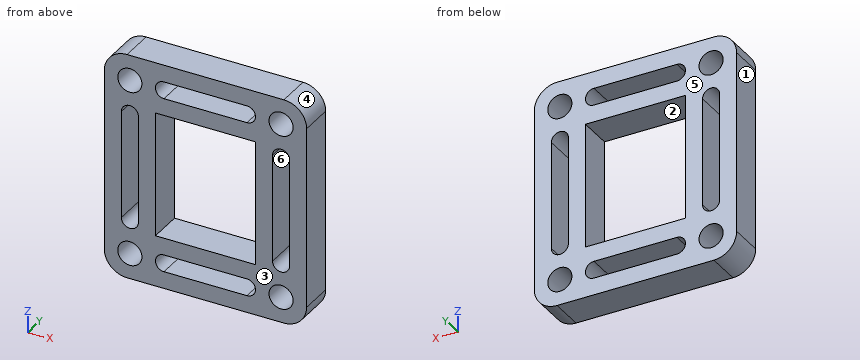
```python
from build123d import *

# Parameters (mm, degrees)
SKETCH1_R           = 2.694076836
SKETCH1_W           = 22.352
SKETCH1_H           = 27.94
BOSS_EXTRUDE1_DEPTH = 7.62


with BuildPart() as part:
    # Sketch1 → Boss-Extrude1 (new body)
    with BuildSketch(Plane(origin=(0, 0, 0), x_dir=(1, 0, 0), z_dir=(0, 1, 0))):
        with BuildLine():
            Line((-22.606, -20.32), (-22.606, 20.32))
            ThreePointArc((-22.606, 20.32), (-21.118102448, 23.912102448), (-17.526, 25.4))
            Line((-17.526, 25.4), (17.526, 25.4))
            ThreePointArc((17.526, 25.4), (21.118102448, 23.912102448), (22.606, 20.32))
            Line((22.606, 20.32), (22.606, -20.32))
            ThreePointArc((22.606, -20.32), (21.118102448, -23.912102448), (17.526, -25.4))
            Line((17.526, -25.4), (-17.526, -25.4))
            ThreePointArc((-17.526, -25.4), (-21.118102448, -23.912102448), (-22.606, -20.32))
        make_face()
        with Locations((16.891, 19.685)):
            Circle(SKETCH1_R, mode=Mode.SUBTRACT)
        with Locations((16.891, -19.685)):
            Circle(SKETCH1_R, mode=Mode.SUBTRACT)
        with Locations((-16.891, -19.685)):
            Circle(SKETCH1_R, mode=Mode.SUBTRACT)
        with Locations((-16.891, 19.685)):
            Circle(SKETCH1_R, mode=Mode.SUBTRACT)
        Rectangle(SKETCH1_W, SKETCH1_H, mode=Mode.SUBTRACT)
        with BuildLine():
            Line((18.796, 12.065), (18.796, -12.065))
            ThreePointArc((18.796, -12.065), (16.891, -13.97), (14.986, -12.065))
            Line((14.986, -12.065), (14.986, 12.065))
            ThreePointArc((14.986, 12.065), (16.891, 13.97), (18.796, 12.065))
        make_face(mode=Mode.SUBTRACT)
        with BuildLine():
            Line((-9.271, -17.78), (9.271, -17.78))
            ThreePointArc((9.271, -17.78), (11.176, -19.685), (9.271, -21.59))
            Line((9.271, -21.59), (-9.271, -21.59))
            ThreePointArc((-9.271, -21.59), (-11.176, -19.685), (-9.271, -17.78))
        make_face(mode=Mode.SUBTRACT)
        with BuildLine():
            Line((-9.271, 17.78), (9.271, 17.78))
            ThreePointArc((9.271, 17.78), (11.176, 19.685), (9.271, 21.59))
            Line((9.271, 21.59), (-9.271, 21.59))
            ThreePointArc((-9.271, 21.59), (-11.176, 19.685), (-9.271, 17.78))
        make_face(mode=Mode.SUBTRACT)
        with BuildLine():
            Line((-18.796, 12.065), (-18.796, -12.065))
            ThreePointArc((-18.796, -12.065), (-16.891, -13.97), (-14.986, -12.065))
            Line((-14.986, -12.065), (-14.986, 12.065))
            ThreePointArc((-14.986, 12.065), (-16.891, 13.97), (-18.796, 12.065))
        make_face(mode=Mode.SUBTRACT)
    extrude(amount=BOSS_EXTRUDE1_DEPTH)


solid = part.part
```
Read the model definition and answer for the solid it produces. Units are mm, in the model's axes. Face numbers are marked on the shaded views. A direction names the side the tool comes from. Give positions to 0.01 mm unless a question says otherwise; leave off trailing zeros. Loops run counter-clockwise (first coordinate to the right, second up) from the corner with the lowest first, then second, coordinate; pieces in that order, holes last.
Item 1: Find the intervals of material crossed by line 1 along X through (y, z) = (7, -2); line 2 along Z through (x, y) = (-2, 0.5); line 3 along X through (y, z) = (2.25, 19.5), in increasing order.
Item 2: This flat-tipped pin is pushed along its axis until it touches: pin 1 Ø8 at (x, z) = (17.5, 5) entering from -Y. Where does it stop, or does it pass through?
Item 3: The part is cut by section C-C (y = 5.25). Give the number of separate pieces and of enclosed holes in the cut face, and give its area (3 significant figures).
Item 4: The mould has two halves that part along X. Classify the marked faces 1, 2, 3 and 4: released by +X, released by -X, zero draft, split by the parting line, or undercut.
Item 5: The part is cut by section B-B (x = -3). Write down the section's boundary in (y, z), and give its area (3 significant figures).
Item 6: For the marked faces 5 and 6, determine the directions among +Z, -Z, +X, -X, +Y, -Y from which every point of the face is accessible in a straight line to the end or side of a thin tool.
Item 7: The part is cut by section A-A (z = -4). Write down the section's boundary in (x, y).
Taken from the geometry:
1. line 1: x = -22.61 to -18.8, -14.99 to -11.18, 11.18 to 14.99, 18.8 to 22.61
1. line 2: z = -25.4 to -21.59, -17.78 to -13.97, 13.97 to 17.78, 21.59 to 25.4
1. line 3: x = -22.61 to -19.58, -14.2 to -11.17, 11.17 to 14.2, 19.58 to 22.61
2. pin 1: stops at y = 0
3. separate pieces: 1
3. enclosed holes: 9
3. area: 1,190 mm2
4. face 1: released by -X
4. face 2: undercut
4. face 3: zero draft
4. face 4: released by +X
5. outline: (0, -25.4) - (7.62, -25.4) - (7.62, -21.59) - (0, -21.59) - close; (0, -17.78) - (7.62, -17.78) - (7.62, -13.97) - (0, -13.97) - close; (0, 13.97) - (7.62, 13.97) - (7.62, 17.78) - (0, 17.78) - close; (0, 21.59) - (7.62, 21.59) - (7.62, 25.4) - (0, 25.4) - close
5. area: 116 mm2
6. face 5: +Z, -Z, +X, -X, +Y
6. face 6: +Y, -Y
7. outline: (-22.61, 0) - (-18.8, 0) - (-18.8, 7.62) - (-22.61, 7.62) - close; (-14.99, 0) - (-11.18, 0) - (-11.18, 7.62) - (-14.99, 7.62) - close; (11.18, 0) - (14.99, 0) - (14.99, 7.62) - (11.18, 7.62) - close; (18.8, 0) - (22.61, 0) - (22.61, 7.62) - (18.8, 7.62) - close
